from build123d import *

# Parameters (mm, degrees)
BOSS_EXTRU_1_DEPTH      = 10
ESQUISSE2_R             = 10
ENL_V_MAT_EXTRU_1_DEPTH = 289.682150945
ENL_V_MAT_EXTRU_2_DEPTH = 289.682150945
ENL_V_MAT_EXTRU_3_DEPTH = 289.682150945
ESQUISSE5_W             = 30
ESQUISSE5_H             = 55
ENL_V_MAT_EXTRU_4_DEPTH = 289.682150945
ESQUISSE6_R             = 1.5
ENL_V_MAT_EXTRU_5_DEPTH = 10
ESQUISSE7_R             = 1.5
ENL_V_MAT_EXTRU_6_DEPTH = 60


with BuildPart() as part:
    # Esquisse1 → Boss.-Extru.1 (new body)
    with BuildSketch(Plane.XY):
        Polygon((-70, 48.885389988), (70, 48.885389988), (70, -31.114610012), (95.621778265, -75.492831747), (164.903810568, -115.492831747), (94.903810568, -236.736388277), (25.621778265, -196.736388277), (-25.621778265, -196.736388277), (-94.903810568, -236.736388277), (-164.903810568, -115.492831747), (-95.621778265, -75.492831747), (-70, -31.114610012), align=None)
    extrude(amount=BOSS_EXTRU_1_DEPTH)

    # Esquisse2 → Enlèv. mat.-Extru.1 (cut, through all)
    with BuildSketch(Plane(origin=(0, 0, 0), x_dir=(-1, 0, 0), z_dir=(0, 0, -1))):
        with Locations((0, -100.541267528)):
            Circle(ESQUISSE2_R)
    extrude(amount=-ENL_V_MAT_EXTRU_1_DEPTH, mode=Mode.SUBTRACT)

    # Esquisse3 → Enlèv. mat.-Extru.2 (cut, through all)
    with BuildSketch(Plane.XY.offset(10)):
        Polygon((-89.77241336, -135.624228955), (-137.403810568, -163.124228955), (-122.403810568, -189.104991068), (-74.77241336, -161.604991068), align=None)
    extrude(amount=-ENL_V_MAT_EXTRU_2_DEPTH, mode=Mode.SUBTRACT)

    # Esquisse4 → Enlèv. mat.-Extru.3 (cut, through all)
    with BuildSketch(Plane.XY.offset(10)):
        Polygon((137.403810568, -163.124228955), (122.403810568, -189.104991068), (74.77241336, -161.604991068), (89.77241336, -135.624228955), align=None)
    extrude(amount=-ENL_V_MAT_EXTRU_3_DEPTH, mode=Mode.SUBTRACT)

    # Esquisse5 → Enlèv. mat.-Extru.4 (cut, through all)
    with BuildSketch(Plane.XY.offset(10)):
        with Locations((0, 21.385389988)):
            Rectangle(ESQUISSE5_W, ESQUISSE5_H)
    extrude(amount=-ENL_V_MAT_EXTRU_4_DEPTH, mode=Mode.SUBTRACT)

    # Esquisse6 → Enlèv. mat.-Extru.5 (cut)
    with BuildSketch(Plane.XY.offset(10)):
        with Locations((-136.848202602, -155.586570181)):
            Circle(ESQUISSE6_R)
        with Locations((-99.609110239, -134.086570181)):
            Circle(ESQUISSE6_R)
        with Locations((-149.848202602, -133.069909683)):
            Circle(ESQUISSE6_R)
        with Locations((-112.609110239, -111.569909683)):
            Circle(ESQUISSE6_R)
    extrude(amount=-ENL_V_MAT_EXTRU_5_DEPTH, mode=Mode.SUBTRACT)

    # Esquisse7 → Enlèv. mat.-Extru.6 (cut)
    with BuildSketch(Plane.XY.offset(10)):
        with Locations((21.25, 44.635389988)):
            Circle(ESQUISSE7_R)
        with Locations((47.25, 44.635389988)):
            Circle(ESQUISSE7_R)
        with Locations((21.25, 1.635389988)):
            Circle(ESQUISSE7_R)
        with Locations((47.25, 1.635389988)):
            Circle(ESQUISSE7_R)
        with Locations((115.598202602, -192.392649842)):
            Circle(ESQUISSE7_R)
        with Locations((78.359110239, -170.892649842)):
            Circle(ESQUISSE7_R)
        with Locations((65.359110239, -193.40931034)):
            Circle(ESQUISSE7_R)
        with Locations((102.598202602, -214.90931034)):
            Circle(ESQUISSE7_R)
    extrude(amount=-ENL_V_MAT_EXTRU_6_DEPTH, mode=Mode.SUBTRACT)


solid = part.part
The model under review builds one solid part; all positions refer to its coordinate system, in mm. A direction names the side the tool comes from. Give positions to 0.01 mm unless a question says otherwise; leave off trailing zeros. Loops run counter-clockwise (first coordinate to the right, second up) from the corner with the lowest first, then second, coordinate; pieces in that order, holes last. Notation, with made-up numbers: (31, 64.25) -> (75, 64.25) arc R17 ccw to (75, 75.25) -> close; hole circle Ø3 at (54.25, 6.5). An arc over 180 degrees is marked (long way). Write each question's results on one line, items separated by ' | '.
1) Take a section at A-A, the plane y = 19. Give the boundary of the cut face in (x, z), plus the area to 3 significant figures.
Conclusion:
outline: (-70, 0) -> (-15, 0) -> (-15, 10) -> (-70, 10) -> close; (15, 0) -> (70, 0) -> (70, 10) -> (15, 10) -> close | area: 1,100 mm^2
2) Tool access review of faces 5 (the face through (82.167, -148.796, 5.07)), 6 (the face through (-70, 8, 5)), 7 (the face through (15, 21, 5)), 8 (the face through (-59.778, -216.456, 4.93)): name each direction out of +Z, -Z, +X, -X, +Y, -Y from which nothing blocks a thin tool from reaching the whole face with its end or side.
Conclusion:
face 5: +Z, -Z | face 6: +Z, -Z, -X, +Y | face 7: +Z, -Z, +Y | face 8: +Z, -Z, -Y
3) Draft analysis for pull direction X (two halves, no side actions). For faces 1 (the face through (2, -124, 0)), 2 (the face through (0, -6.115, 5)), 3 (the face through (-82.167, -148.796, 5.07)), 4 (the face through (151.346, -138.975, 4.93)), state which applies: pulls with the +X half, pulls with the -X half, needs draft (parallel to the pull), parting line crosses it, or undercut.
Conclusion:
face 1: needs draft | face 2: undercut | face 3: undercut | face 4: pulls with the +X half
4) Take a section at B-B, the plane x = 0. Give the boundary of the cut face in (y, z), plus the area to 3 significant figures.
Conclusion:
outline: (-196.74, 0) -> (-110.54, 0) -> (-110.54, 10) -> (-196.74, 10) -> close; (-90.54, 0) -> (-6.11, 0) -> (-6.11, 10) -> (-90.54, 10) -> close | area: 1,710 mm^2
5) Insertion check: pin 1 Ø3 at (x, z) = (6, 7) entering from +Y; pin 2 Ø2 at (y, z) = (-32.5, 8.5) entering from +X; pin 3 Ø1.5 at (x, z) = (86.5, 3.5) entering from -Y. Each pin has a flat end and moves straight along its axis. Give the tip position at first contact, or say it passes through.
Conclusion:
pin 1: stops at y = -6.11 | pin 2: stops at x = 71.38 | pin 3: stops at y = -232.32
6) Take a section at C-C, the plane y = -16. Give the boundary of the cut face in (x, z).
Conclusion:
outline: (-70, 0) -> (70, 0) -> (70, 10) -> (-70, 10) -> close
7) Take a section at D-D, the plane z = 2.75. Count the separate pieces of the cut face and the enclosed holes in it, plus the area to 3 significant figures.
Conclusion:
separate pieces: 1 | enclosed holes: 13 | area: 50,300 mm^2
8) For line 1 along X through (y, z) = (30, 5.5); line 2 along X through (y, z) = (-139, 4.25); line 3 along Y through (x, z) = (20, 6.5), list the stretches that pass through material, from the lowest coordinate up. Write a range as from..to.
Conclusion:
line 1: x = -70..-15, 15..70 | line 2: x = -151.33..-95.62, -87.82..87.82, 95.62..151.33 | line 3: y = -196.74..0.81, 2.46..43.81, 45.46..48.89
